Verification items for this drawing (mm, ordinates from the low corner). Coordinates: 2 decimals unless noted, no trailing zeros. Write each loop counter-clockwise with the first axis right and the second up, starting at its lowest first coordinate (ties: lowest second). Pieces come first, ordered by that corner, then holes. Notation, with made-up numbers: M -38,-18 L -1,-18 A10 ccw -1,-6 Z; hole C 9.25,38 d10. An arc over 180 degrees is marked long. Write each question's results on one line, items separated by ' | '.
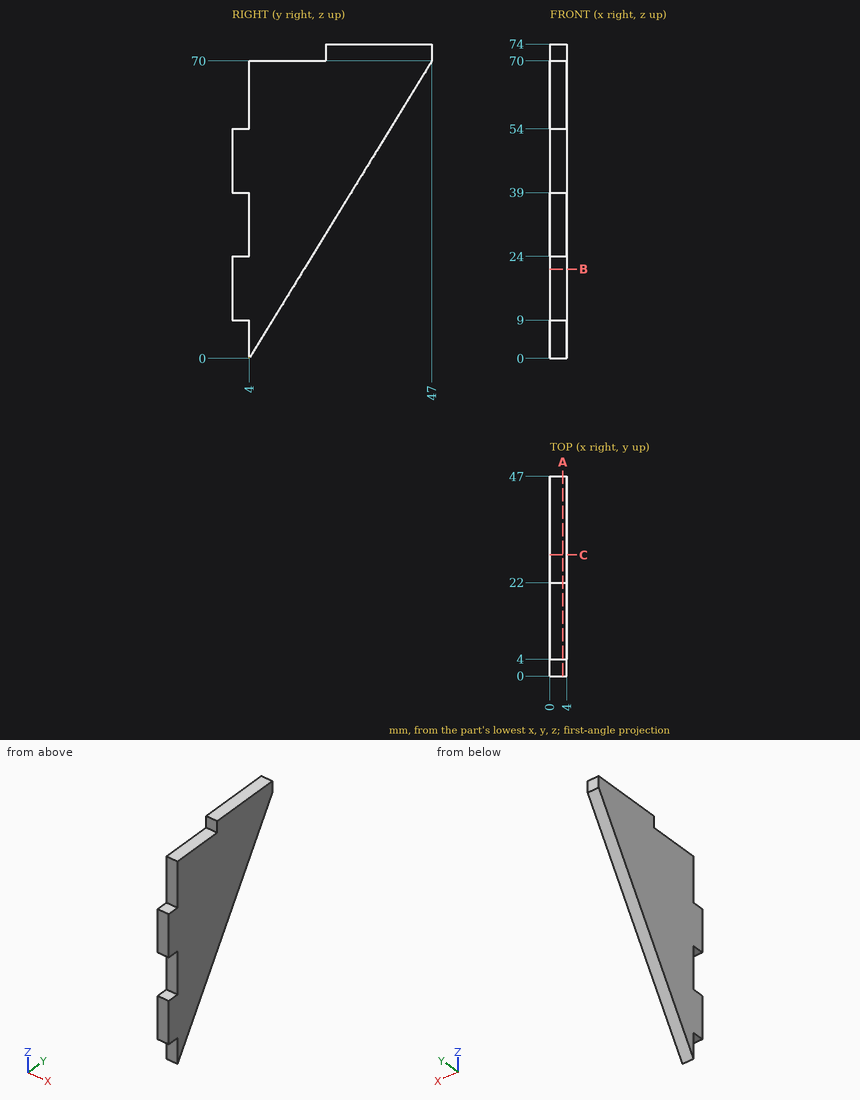
Q1. Sectioned sample at A-A on x = 3.1. Record the cut outline in (y, z).
Geometry check:
outline: M 0,9 L 4,9 L 4,0 L 47,70 L 47,74 L 22,74 L 22,70 L 4,70 L 4,54 L 0,54 L 0,39 L 4,39 L 4,24 L 0,24 Z
Q2. Sectioned sample at C-C on y = 28.5. Record the cut outline in (x, z).
Geometry check:
outline: M 0,39.88 L 4,39.88 L 4,74 L 0,74 Z
Q3. Depth check by flat-ended pin: P1, Ø1.2, axis at x = 1, y = 2, coming from the -Z side; P2, Ø1.2, axis at x = 2, z = 72.5, coming from the -Y side; P3, Ø2, axis at x = 2, z = 32.5, coming from the -Y side. Enter the tip coordinate at first touch or a pass-through.
Geometry check:
P1: stops at z = 9 | P2: stops at y = 22 | P3: stops at y = 4
Q4. Scan lines: probe 1 along Z at (x, y) = (1.65, 18.5); probe 2 along Y at (x, z) = (2.55, 36); probe 3 along Z at (x, y) = (2.3, 37). Record each from-to range of solid material in increasing order.
Geometry check:
probe 1: z = 23.6 to 70 | probe 2: y = 4 to 26.11 | probe 3: z = 53.72 to 74
Q5. Sectioned sample at B-B on z = 21. Record the cut outline in (x, y), and give its area (3 significant figures).
Geometry check:
outline: M 0,0 L 4,0 L 4,16.9 L 0,16.9 Z | area: 67.6 mm2
